Build history of the part. All positions in model axes, mm. Coordinates: 2 decimals unless noted, no trailing zeros. Write each question's results on one line, items separated by ' | '.
from build123d import *

# Parameters (mm, degrees)
BOSS_EXTRUDE1_DEPTH   = 710
SKETCH3_R             = 3.4
CUT_EXTRUDE1_DEPTH    = 716.611626513
CUT_EXTRUDE2_DEPTH    = 716.611626513
FILLET1_R             = 1
FILLET2_R             = 1
FILLET3_R             = 1
CUT_EXTRUDE3_DEPTH    = 716.611626513
CUT_EXTRUDE4_DEPTH    = 716.611626513
FILLET4_R             = 1
FILLET5_R             = 1
FILLET6_R             = 1
FILLET7_R             = 1
FILLET8_R             = 1
FILLET9_R             = 1
FILLET10_R            = 1
FILLET11_R            = 1
MIRROR11_COPY_1_DEPTH = 716.611626513
MIRROR11_COPY_2_DEPTH = 716.611626513
CUT_EXTRUDE5_DEPTH    = 1000


with BuildPart() as part:
    # Sketch1 → Boss-Extrude1 (new body)
    with BuildSketch(Plane(origin=(0, 0, 0), x_dir=(1, 0, 0), z_dir=(0, 1, 0))):
        with BuildLine():
            Line((5, 0), (75, 0))
            ThreePointArc((75, 0), (78.535533906, -1.464466094), (80, -5))
            Line((80, -5), (80, -35))
            ThreePointArc((80, -35), (78.535533906, -38.535533906), (75, -40))
            Line((75, -40), (5, -40))
            ThreePointArc((5, -40), (1.464466094, -38.535533906), (0, -35))
            Line((0, -35), (0, -5))
            ThreePointArc((0, -5), (1.464466094, -1.464466094), (5, 0))
        make_face()
    extrude(amount=BOSS_EXTRUDE1_DEPTH)

    # Sketch3 → Cut-Extrude1 (cut, through all)
    with BuildSketch(Plane(origin=(0, 710, 0), x_dir=(1, 0, 0), z_dir=(0, 1, 0))):
        with Locations(Location((20, -20, 0), (0, 0, 270))):
            Circle(SKETCH3_R)
    cut_extrude1 = extrude(amount=-CUT_EXTRUDE1_DEPTH, mode=Mode.SUBTRACT)

    # Mirror3: Cut-Extrude1 across plane
    add(cut_extrude1.mirror(Plane(origin=(40, 0, 0), x_dir=(0, 0, 1), z_dir=(1, 0, 0))), mode=Mode.SUBTRACT)

    # Sketch7 → Cut-Extrude2 (cut, symmetric)
    with BuildSketch(Plane(origin=(0, 0, 0), x_dir=(-1, 0, 0), z_dir=(0, -1, 0))):
        with BuildLine():
            Line((-15.9, -40), (-24.1, -40))
            Line((-24.1, -40), (-24.1, -36.5))
            ThreePointArc((-24.1, -36.5), (-24.392893219, -35.792893219), (-25.1, -35.5))
            Line((-25.1, -35.5), (-29.489753594, -35.5))
            ThreePointArc((-29.489753594, -35.5), (-30.415270825, -34.8787055), (-30.190750526, -33.786835712))
            Line((-30.190750526, -33.786835712), (-24.391814382, -28.086835712))
            ThreePointArc((-24.391814382, -28.086835712), (-24.069522951, -27.874482769), (-23.69081745, -27.8))
            Line((-23.69081745, -27.8), (-16.309186536, -27.8))
            ThreePointArc((-16.309186536, -27.8), (-15.930477876, -27.874484063), (-15.608184734, -28.086840499))
            Line((-15.608184734, -28.086840499), (-9.809327805, -33.786840499))
            ThreePointArc((-9.809327805, -33.786840499), (-9.584813669, -34.87870866), (-10.510329607, -35.5))
            Line((-10.510329607, -35.5), (-14.9, -35.5))
            ThreePointArc((-14.9, -35.5), (-15.607106781, -35.792893219), (-15.9, -36.5))
            Line((-15.9, -36.5), (-15.9, -40))
        make_face()
    cut_extrude2 = extrude(amount=CUT_EXTRUDE2_DEPTH, both=True, mode=Mode.SUBTRACT)

    # Fillet1
    fillet1_edges = [part.edges().sort_by_distance(p)[0] for p in [
        (15.9, 355, 40),
        (24.1, 355, 40),
    ]]
    fillet(fillet1_edges, radius=FILLET1_R)

    # Mirror8: Cut-Extrude2 across plane
    add(cut_extrude2.mirror(Plane(origin=(40, 0, 0), x_dir=(0, 0, 1), z_dir=(1, 0, 0))), mode=Mode.SUBTRACT)

    # Fillet2
    fillet2_edges = [part.edges().sort_by_distance(p)[0] for p in [
        (55.9, 355, 40),
    ]]
    fillet(fillet2_edges, radius=FILLET2_R)

    # Fillet3
    fillet3_edges = [part.edges().sort_by_distance(p)[0] for p in [
        (64.1, 355, 40),
    ]]
    fillet(fillet3_edges, radius=FILLET3_R)

    # Sketch9 → Cut-Extrude3 (cut, through all)
    with BuildSketch(Plane(origin=(0, 0, 0), x_dir=(1, 0, 0), z_dir=(0, 1, 0))):
        with BuildLine():
            Line((14.899846923, -4.500713815), (10.450461284, -4.500713815))
            ThreePointArc((10.450461284, -4.500713815), (9.526581751, -5.118030383), (9.743354502, -6.207820596))
            Line((9.743354502, -6.207820596), (15.442640687, -11.907106781))
            ThreePointArc((15.442640687, -11.907106781), (15.767064036, -12.123879533), (16.149747468, -12.2))
            Line((16.149747468, -12.2), (23.850252532, -12.2))
            ThreePointArc((23.850252532, -12.2), (24.232935964, -12.123879533), (24.557359313, -11.907106781))
            Line((24.557359313, -11.907106781), (30.257359313, -6.207106781))
            ThreePointArc((30.257359313, -6.207106781), (30.474132064, -5.117316568), (29.550252532, -4.5))
            Line((29.550252532, -4.5), (25.099846964, -4.5))
            ThreePointArc((25.099846964, -4.5), (24.392724723, -4.207091321), (24.099846965, -3.499956273))
            Line((24.099846965, -3.499956273), (24.100000008, 0))
            Line((24.100000008, 0), (15.9, 0))
            Line((15.9, 0), (15.899846922, -3.500757542))
            ThreePointArc((15.899846922, -3.500757542), (15.606938244, -4.207836056), (14.899846923, -4.500713815))
        make_face()
    cut_extrude3 = extrude(amount=CUT_EXTRUDE3_DEPTH, mode=Mode.SUBTRACT)

    # Mirror9: Cut-Extrude3 across plane
    add(cut_extrude3.mirror(Plane(origin=(40, 0, 0), x_dir=(0, 0, 1), z_dir=(1, 0, 0))), mode=Mode.SUBTRACT)

    # Sketch10 → Cut-Extrude4 (cut, through all)
    with BuildSketch(Plane(origin=(0, 0, 0), x_dir=(1, 0, 0), z_dir=(0, 1, 0))):
        with BuildLine():
            Line((4.5, -14.9), (4.5, -10.58605332))
            ThreePointArc((4.5, -10.58605332), (5.126159695, -9.658560233), (6.220486853, -9.892584724))
            Line((6.220486853, -9.892584724), (11.920486853, -15.814662646))
            ThreePointArc((11.920486853, -15.814662646), (12.127493087, -16.134290938), (12.2, -16.508131242))
            Line((12.2, -16.508131242), (12.2, -23.491868758))
            ThreePointArc((12.2, -23.491868758), (12.127493087, -23.865709062), (11.920486853, -24.185337354))
            Line((11.920486853, -24.185337354), (6.220486853, -30.107415276))
            ThreePointArc((6.220486853, -30.107415276), (5.126159695, -30.341439767), (4.5, -29.41394668))
            Line((4.5, -29.41394668), (4.5, -25.1))
            ThreePointArc((4.5, -25.1), (4.207106781, -24.392893219), (3.5, -24.1))
            Line((3.5, -24.1), (0, -24.1))
            Line((0, -24.1), (0, -15.9))
            Line((0, -15.9), (3.5, -15.9))
            ThreePointArc((3.5, -15.9), (4.207106781, -15.607106781), (4.5, -14.9))
        make_face()
    cut_extrude4 = extrude(amount=CUT_EXTRUDE4_DEPTH, mode=Mode.SUBTRACT)

    # Fillet4
    fillet4_edges = [part.edges().sort_by_distance(p)[0] for p in [
        (24.100000008, 355, 0),
    ]]
    fillet(fillet4_edges, radius=FILLET4_R)

    # Fillet5
    fillet5_edges = [part.edges().sort_by_distance(p)[0] for p in [
        (64.1, 355, 0),
    ]]
    fillet(fillet5_edges, radius=FILLET5_R)

    # Fillet6
    fillet6_edges = [part.edges().sort_by_distance(p)[0] for p in [
        (55.899999992, 355, 0),
    ]]
    fillet(fillet6_edges, radius=FILLET6_R)

    # Fillet7
    fillet7_edges = [part.edges().sort_by_distance(p)[0] for p in [
        (15.9, 355, 0),
    ]]
    fillet(fillet7_edges, radius=FILLET7_R)

    # Fillet8
    fillet8_edges = [part.edges().sort_by_distance(p)[0] for p in [
        (0, 355, 24.1),
    ]]
    fillet(fillet8_edges, radius=FILLET8_R)

    # Fillet9
    fillet9_edges = [part.edges().sort_by_distance(p)[0] for p in [
        (0, 355, 15.9),
    ]]
    fillet(fillet9_edges, radius=FILLET9_R)

    # Mirror10: Cut-Extrude4 across plane
    add(cut_extrude4.mirror(Plane(origin=(40, 0, 0), x_dir=(0, 0, 1), z_dir=(1, 0, 0))), mode=Mode.SUBTRACT)

    # Fillet10
    fillet10_edges = [part.edges().sort_by_distance(p)[0] for p in [
        (80, 355, 15.9),
    ]]
    fillet(fillet10_edges, radius=FILLET10_R)

    # Fillet11
    fillet11_edges = [part.edges().sort_by_distance(p)[0] for p in [
        (80, 355, 24.1),
    ]]
    fillet(fillet11_edges, radius=FILLET11_R)

    # Mirror11 copy 1 sketch → Mirror11 copy 1 (cut, through all)
    with BuildSketch(Plane(origin=(40, 0, 0), x_dir=(1, 0, 0), z_dir=(0, 1, 0))):
        with BuildLine():
            Line((4.5, -14.9), (4.5, -10.58605332))
            ThreePointArc((4.5, -10.58605332), (5.126159695, -9.658560233), (6.220486853, -9.892584724))
            Line((6.220486853, -9.892584724), (11.920486853, -15.814662646))
            ThreePointArc((11.920486853, -15.814662646), (12.127493087, -16.134290938), (12.2, -16.508131242))
            Line((12.2, -16.508131242), (12.2, -23.491868758))
            ThreePointArc((12.2, -23.491868758), (12.127493087, -23.865709062), (11.920486853, -24.185337354))
            Line((11.920486853, -24.185337354), (6.220486853, -30.107415276))
            ThreePointArc((6.220486853, -30.107415276), (5.126159695, -30.341439767), (4.5, -29.41394668))
            Line((4.5, -29.41394668), (4.5, -25.1))
            ThreePointArc((4.5, -25.1), (4.207106781, -24.392893219), (3.5, -24.1))
            Line((3.5, -24.1), (0, -24.1))
            Line((0, -24.1), (0, -15.9))
            Line((0, -15.9), (3.5, -15.9))
            ThreePointArc((3.5, -15.9), (4.207106781, -15.607106781), (4.5, -14.9))
        make_face()
    extrude(amount=MIRROR11_COPY_1_DEPTH, mode=Mode.SUBTRACT)

    # Mirror11 copy 2 sketch → Mirror11 copy 2 (cut, through all)
    with BuildSketch(Plane(origin=(120, 0, 0), x_dir=(-1, 0, 0), z_dir=(0, 1, 0))):
        with BuildLine():
            Line((4.5, 14.9), (4.5, 10.58605332))
            ThreePointArc((4.5, 10.58605332), (5.126159695, 9.658560233), (6.220486853, 9.892584724))
            Line((6.220486853, 9.892584724), (11.920486853, 15.814662646))
            ThreePointArc((11.920486853, 15.814662646), (12.127493087, 16.134290938), (12.2, 16.508131242))
            Line((12.2, 16.508131242), (12.2, 23.491868758))
            ThreePointArc((12.2, 23.491868758), (12.127493087, 23.865709062), (11.920486853, 24.185337354))
            Line((11.920486853, 24.185337354), (6.220486853, 30.107415276))
            ThreePointArc((6.220486853, 30.107415276), (5.126159695, 30.341439767), (4.5, 29.41394668))
            Line((4.5, 29.41394668), (4.5, 25.1))
            ThreePointArc((4.5, 25.1), (4.207106781, 24.392893219), (3.5, 24.1))
            Line((3.5, 24.1), (0, 24.1))
            Line((0, 24.1), (0, 15.9))
            Line((0, 15.9), (3.5, 15.9))
            ThreePointArc((3.5, 15.9), (4.207106781, 15.607106781), (4.5, 14.9))
        make_face()
    extrude(amount=MIRROR11_COPY_2_DEPTH, mode=Mode.SUBTRACT)

    # Mirror12: Cut-Extrude4 across plane
    add(cut_extrude4.mirror(Plane.ZY.offset(-20)), mode=Mode.SUBTRACT)

    # Sketch12 → Cut-Extrude5 (cut)
    with BuildSketch(Plane(origin=(0, 0, 0), x_dir=(-1, 0, 0), z_dir=(0, -1, 0))):
        with BuildLine():
            Line((-28.079513147, -24.185337354), (-39.327067998, -35.871108628))
            ThreePointArc((-39.327067998, -35.871108628), (-40.049082116, -36.177638866), (-40.770156561, -35.868904648))
            Line((-40.770156561, -35.868904648), (-51.922601709, -24.210885791))
            ThreePointArc((-51.922601709, -24.210885791), (-52.128062958, -23.892044517), (-52.2, -23.519621175))
            Line((-52.2, -23.519621175), (-52.2, -16.508131242))
            ThreePointArc((-52.2, -16.508131242), (-52.127493087, -16.134290938), (-51.920486853, -15.814662646))
            Line((-51.920486853, -15.814662646), (-40.720486853, -4.17829901))
            ThreePointArc((-40.720486853, -4.17829901), (-40, -3.871767606), (-39.279513147, -4.17829901))
            Line((-39.279513147, -4.17829901), (-28.079513147, -15.814662646))
            ThreePointArc((-28.079513147, -15.814662646), (-27.872506913, -16.134290938), (-27.8, -16.508131242))
            Line((-27.8, -16.508131242), (-27.8, -23.491868758))
            ThreePointArc((-27.8, -23.491868758), (-27.872506913, -23.865709062), (-28.079513147, -24.185337354))
        make_face()
    extrude(amount=-CUT_EXTRUDE5_DEPTH, mode=Mode.SUBTRACT)


solid = part.part
1. Band-saw the part on A-A on y = 156.5. Give the number of separate pieces and of enclosed holes in the cut face, then the cut area to 3 significant figures.
Solved:
separate pieces: 1 | enclosed holes: 3 | area: 1,660 mm2
2. Two-plate mould, pull along X, no slides. Class faces 1 (the face through (49, 710, 11)), 2 (the face through (46.27, 350.03, 30.12)): +X half, -X half, draft (parallel to the pull), parting line (faces both ways), or undercut.
Solved:
face 1: draft | face 2: undercut
3. Drop flat-ended pins along their axis: pin 1 Ø2 at (x, y) = (2.5, 317.5) entering from +Z; pin 2 Ø2 at (x, z) = (49.5, 13.5) entering from +Y; pin 3 Ø3.5 at (y, z) = (283, 19) entering from +X; pin 4 Ø3 at (y, z) = (395.5, 37.5) entering from -X. Give the stop position or say it passes through.
Solved:
pin 1: stops at z = 39.77 | pin 2: stops at y = 710 | pin 3: stops at x = 67.8 | pin 4: stops at x = 0.1
4. Probe line 1 (X direction, y = 481, z = 20); line 2 (Z direction, x = 53.5, y = 382.5); line 3 (Z direction, x = 13, y = 181.5). List the from-to ranges inside material, lowest first.
Solved:
line 1: x = 12.2 to 16.6, 23.4 to 27.8, 52.2 to 56.6, 63.4 to 67.8 | line 2: z = 0 to 4.5, 9.96 to 30.16, 35.5 to 40 | line 3: z = 0 to 4.5, 9.46 to 30.65, 35.5 to 40
